Could you check a few things on this model? Use its own coordinates, in mm. Face numbers are marked on the shaded views. Coordinates: 2 decimals unless noted, no trailing zeros. Order: outer loops, then holes, each group sorted by start corner. A loop starts at its lowest first (then second) coordinate and runs counter-clockwise, first axis right, second up. Notation, with made-up numbers: (38.25, -15.75) -> (60.25, -15.75) arc R27 cw to (60.25, 1.25) -> close; hole circle Ø6 at (-7.75, 0). An arc over 180 degrees is marked (long way). Put each result on its own line as item: value. Start each with the question number.
Q1. Will these pins go through, and if not, where does the flat tip stop? pin 1 (2 mm diameter, centred on x = 235, y = -6, fed in from +Z); pin 2 (1 mm diameter, centred on y = -2, z = 31.5, fed in from +X); pin 3 (8 mm diameter, centred on y = -17, z = 38.5, fed in from -X).
Q2. Please list where these lines run through material, in increasing order: line 1 along Y through (x, z) = (233.25, 35); line 2 along Y through (x, z) = (231.25, 43); line 3 along Z through (x, y) = (233.25, -20).
Q3. We'd pull the mould along Y, two halves only. Please class the marked faces 1, 2 and 3: +Y half, -Y half, draft (parallel to the pull), parting line (faces both ways), or undercut.
Q4. If we section it at D-D (z = 38): Please give me the cut outline in (x, y), and give its area (3 significant figures).
Q5. If we section it at B-B (y = -19.5): Count the separate pieces of the cut face and the enclosed holes in it, and give its area (3 significant figures).
Q6. If we section it at A-A (z = 48): Please give me the cut outline in (x, y).
from build123d import *

# Parameters (mm, degrees)
SKETCH1_R           = 14.9606
BOSS_EXTRUDE1_DEPTH = 6.35
SKETCH2_R           = 2.54
CUT_EXTRUDE1_DEPTH  = 6.35
SKETCH3_R           = 1.5875
CUT_EXTRUDE2_DEPTH  = 10
SKETCH5_R           = 15.875
SKETCH5_R_2         = 14.9606
BOSS_EXTRUDE2_DEPTH = 3.175


with BuildPart() as part:
    # Sketch1 → Boss-Extrude1 (new body)
    with BuildSketch(Plane(origin=(234.278878836, -18.689027227, 0), x_dir=(0, 0, -1), z_dir=(0.9968332748770866, -0.0795199477981641, 0))):
        with Locations(Location((-43.174261814, 8.550344032, 0), (0, 0, 90))):
            Circle(SKETCH1_R)
    extrude(amount=-BOSS_EXTRUDE1_DEPTH)

    # Sketch2 → Cut-Extrude1 (cut)
    with BuildSketch(Plane(origin=(234.278878836, -18.689027227, 0), x_dir=(0, 0, -1), z_dir=(0.9968332748770866, -0.07951994779816411, 0))):
        with Locations(Location((-43.174261814, 8.550344032, 0), (0, 0, 90))):
            Circle(SKETCH2_R)
    extrude(amount=-CUT_EXTRUDE1_DEPTH, mode=Mode.SUBTRACT)

    # Sketch3 → Cut-Extrude2 (cut)
    with BuildSketch(Plane(origin=(227.94898754, -18.184075559, 0), x_dir=(0, 0, 1), z_dir=(-0.9968332748770866, 0.07951994779816411, 0))):
        with Locations(Location((30.474261814, 8.550344032, 0), (0, 0, 270))):
            Circle(SKETCH3_R)
        with Locations(Location((43.174261814, 21.250344032, 0), (0, 0, 270))):
            Circle(SKETCH3_R)
        with Locations(Location((52.154517935, 17.530600153, 0), (0, 0, 270))):
            Circle(SKETCH3_R)
        with Locations(Location((55.874261814, 8.550344032, 0), (0, 0, 270))):
            Circle(SKETCH3_R)
        with Locations(Location((52.154517935, -0.429912089, 0), (0, 0, 270))):
            Circle(SKETCH3_R)
        with Locations(Location((43.174261814, -4.149655968, 0), (0, 0, 270))):
            Circle(SKETCH3_R)
        with Locations(Location((34.194005693, -0.429912089, 0), (0, 0, 270))):
            Circle(SKETCH3_R)
        with Locations(Location((34.194005693, 17.530600153, 0), (0, 0, 270))):
            Circle(SKETCH3_R)
    extrude(amount=-CUT_EXTRUDE2_DEPTH, mode=Mode.SUBTRACT)

    # Sketch5 → Boss-Extrude2 (add)
    with BuildSketch(Plane(origin=(234.278878836, -18.689027227, 0), x_dir=(0, 0, 1), z_dir=(-0.9968332748770866, 0.07951994779816411, 0))):
        with Locations(Location((43.174261814, 8.550344032, 0), (0, 0, 270))):
            Circle(SKETCH5_R)
        with Locations(Location((43.174261814, 8.550344032, 0), (0, 0, 90))):
            Circle(SKETCH5_R_2, mode=Mode.SUBTRACT)
    extrude(amount=BOSS_EXTRUDE2_DEPTH)


solid = part.part
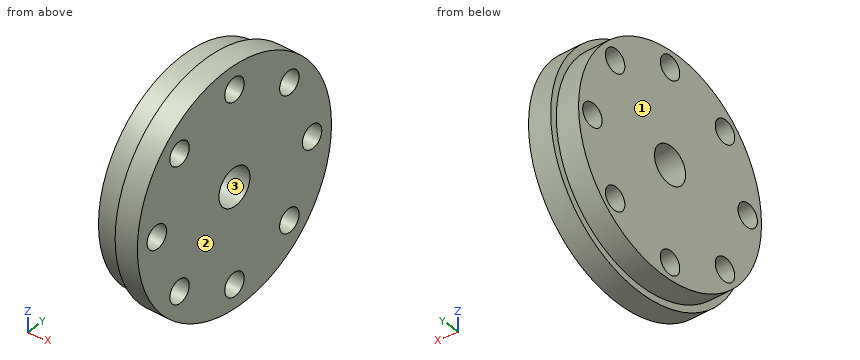
The answers:
1. pin 1: z = 58.73
1. pin 2: x = 235.65
1. pin 3: x = 227.72
2. line 1: -23.68 to -20.41, -17.67 to -2.39, 0.35 to 3.62
2. line 2: -25.79 to -24.19, -21.03 to -12.41, -7.33 to 1.29, 4.45 to 5.14
2. line 3: 30.8 to 32.93, 35.46 to 50.89, 53.42 to 55.55
3. face 1: +Y half
3. face 2: -Y half
3. face 3: undercut
4. outline: (227.51, -23.65) -> (230.68, -23.91) -> (230.6, -24.87) -> (233.77, -25.13) -> (236.15, 4.79) -> (232.99, 5.05) -> (232.91, 4.08) -> (229.75, 4.33) -> close
4. area: 184 mm^2
5. separate pieces: 3
5. enclosed holes: 0
5. area: 117 mm^2
6. outline: (227.5, -23.78) -> (230.67, -24.03) -> (230.59, -24.99) -> (233.76, -25.24) -> (236.16, 4.91) -> (233, 5.16) -> (232.92, 4.2) -> (229.75, 4.46) -> close
